from build123d import *

# Parameters (mm, degrees)
SKETCH1_R           = 2.675
BOSS_EXTRUDE1_DEPTH = 4.5
BOSS_EXTRUDE2_DEPTH = 3


with BuildPart() as part:
    # Sketch1 → Boss-Extrude1 (new body)
    with BuildSketch(Plane.XY):
        with BuildLine():
            Line((1.335499014, 8.518725494), (1.335499014, -16.481274506))
            ThreePointArc((1.335499014, -16.481274506), (2.213885401, -17.473852024), (3.305919272, -16.722696381))
            Line((3.305919272, -16.722696381), (7.593768545, 0.512758361))
            ThreePointArc((7.593768545, 0.512758361), (16.08527887, 13.599607486), (1.335499014, 8.518725494))
        make_face()
        with Locations((9.585499014, 6.518725494)):
            Circle(SKETCH1_R, mode=Mode.SUBTRACT)
    extrude(amount=BOSS_EXTRUDE1_DEPTH)

    # Sketch2 → Boss-Extrude2 (add)
    with BuildSketch(Plane.XY.offset(4.5)):
        with BuildLine():
            Line((1.335499014, -13.503541952), (1.335499014, -16.481274506))
            ThreePointArc((1.335499014, -16.481274506), (2.213885401, -17.473852024), (3.305919272, -16.722696381))
            Line((3.305919272, -16.722696381), (4.024809049, -13.833044386))
            ThreePointArc((4.024809049, -13.833044386), (2.866323075, -12.148831621), (1.335499014, -13.503541952))
        make_face()
    extrude(amount=BOSS_EXTRUDE2_DEPTH)


solid = part.part
Source: CAD feature listing. Evaluate the final solid. Frame: model axes, mm. Coordinates: 2 decimals unless noted, no trailing zeros. Loops run counter-clockwise (first coordinate to the right, second up) from the corner with the lowest first, then second, coordinate; pieces in that order, holes last. Notation, with made-up numbers: (50, 64) -> (77, 64) arc R18 ccw to (77, 96) -> close; hole circle Ø3 at (47, 33.5). An arc over 180 degrees is marked (long way). Answer in a Markdown table with one row per item. Add a question column.
Q1. Ray query, line 1 along Z through (x, y) = (12, 3); line 2 along Y through (x, z) = (8, 3.5); line 3 along X through (y, z) = (-8, 4.25). Return the intervals inside material, ascending.
Q2. Section A-A on x = 8. Return the cut outline in (y, z).
Q3. Contact query for flat-ended pins moving along their axis: pin 1 Ø7 at (x, y) = (9.59, 6.52) entering from +Z; pin 2 Ø3 at (x, z) = (7, 2) entering from +Y; pin 3 Ø1.5 at (x, y) = (11.5, -2) entering from -Z; pin 4 Ø4 at (y, z) = (2, 6) entering from +X. Output: stop coordinate, or through.
Q4. Pull-direction query (Y, two-part tool) for faces 1 (the face through (7.614, 8.327, 2.218)), 2 (the face through (3, -15, 7.5)), 3 (the face through (16.26, 13.37, 2.22)); classes: pulls with the +Y half, pulls with the -Y half, needs draft (parallel to the pull), parting line crosses it, or undercut.
Q5. Section B-B on y = 7. Return the cut outline in (x, z).
Q6. Section D-D on y = -15. Return the cut outline in (x, z), and give its area (3 significant figures).
Computed values:
| question | item | result |
|---|---|---|
| 1 | line 1 | z = 0 to 4.5 |
| 1 | line 2 | y = 0.42 to 4.36, 8.67 to 16.61 |
| 1 | line 3 | x = 1.34 to 5.48 |
| 2 | outline | (0.42, 0) -> (4.36, 0) -> (4.36, 4.5) -> (0.42, 4.5) -> close; (8.67, 0) -> (16.61, 0) -> (16.61, 4.5) -> (8.67, 4.5) -> close |
| 3 | pin 1 | stops at z = 4.5 |
| 3 | pin 2 | stops at y = 16.7 |
| 3 | pin 3 | passes through |
| 3 | pin 4 | stops at x = 15.99 |
| 4 | face 1 | undercut |
| 4 | face 2 | needs draft |
| 4 | face 3 | parting line crosses it |
| 5 | outline | (1.34, 0) -> (6.95, 0) -> (6.95, 4.5) -> (1.34, 4.5) -> close; (12.22, 0) -> (17.69, 0) -> (17.69, 4.5) -> (12.22, 4.5) -> close |
| 6 | outline | (1.34, 0) -> (3.73, 0) -> (3.73, 7.5) -> (1.34, 7.5) -> close |
| 6 | area | 18.0 mm^2 |
